Geometry: final body of the model. Coordinates: model frame, mm. A direction names the side the tool comes from. Give positions to 0.01 mm unless a question says otherwise; leave off trailing zeros. Write each loop counter-clockwise with the first axis right and the second up, starting at its lowest first coordinate (ties: lowest second). Pieces come first, ordered by that corner, then holes. Notation, with made-up numbers: M -7.75,71 L 42.25,71 A9 ccw 42.25,88 Z; hole C -18.5,5 d10. An arc over 180 degrees is marked long. Use a Markdown table: item, result. Add a question column.
(1) Draft query along X for faces 1 (the flat face through (24, 0, -25)), 2 (the flat face through (24, 14, -58)), 3 (the flat face through (-10, 13, -26)). Return one class per face: released by +X, released by -X, zero draft, split by the parting line, or undercut.
(2) Cut plane A-A (y = 24). Output: boundary loops of the cut face in (x, z), plus the area to 3 significant figures.
(3) Reachability of faces 4 (the flat face through (24, 13, -59)), 5 (the flat face through (23, 14, 7)) from +Z, -Z, +X, -X, +Y, -Y: full face, straight path, thin tool, end or side. Return the list, or none.
(4) Material intervals for L1, parallel to X at y = 4.5, z = -4.5; L2, parallel to Z at x = 45, y = 18; L3, parallel to Y at x = 19.5, z = -28, sorted ascending.
(5) Cut plane B-B (x = 29.5). Output: boundary loops of the cut face in (y, z), plus the area to 3 significant figures.
(6) Cut plane D-D (z = -8). Output: boundary loops of the cut face in (x, y), plus the area to 3 significant figures.
(7) Cut plane C-C (x = -3). Output: boundary loops of the cut face in (y, z), plus the area to 3 significant figures.
Autodesk Inventor part; units mm, degrees
ref_plane "YZ Plane" through (0, 0, 0) normal (1, 0, 0) x (0, 1, 0)
ref_plane "XZ Plane" through (0, 0, 0) normal (0, 1, 0) x (-1, 0, 0)
ref_plane "XY Plane" through (0, 0, 0) normal (0, 0, 1) x (1, 0, 0)
sketch "Boceto1" plane through (0, 0, 0) normal (0, 1, 0) x (-1, 0, 0)
  line L0 (9, 7) -> (-56, 7)
  line L1 (-56, 7) -> (-56, -58)
  line L2 (-56, -58) -> (9, -58)
  line L3 (9, -58) -> (9, 7)
  point P0 (0, 0)
  dimension "d0" = 65
  dimension "d1" = 65
extrude "Extrusión1" add sketch "Boceto1" along normal blind 3
sketch "Boceto2" plane through (0, 3, 0) normal (0, 1, 0) x (1, 0, 0)
  line L0 (-9, -7) -> (56, -7)
  line L1 (56, -7) -> (56, 58)
  line L2 (56, 58) -> (-9, 58)
  line L3 (-9, 58) -> (-9, -7)
  line L4 (-10, -8) -> (57, -8)
  line L5 (57, -8) -> (57, 59)
  line L6 (57, 59) -> (-10, 59)
  line L7 (-10, 59) -> (-10, -8)
  line L8 (-10, -8) -> (57, 59) construction
  line L9 (57, -8) -> (-10, 59) construction
  point P0 (0, 0)
  point P1 (23.5, 25.5)
  dimension "d4" = 67
  dimension "d5" = 67
extrude "Extrusión2" add sketch "Boceto2" against normal blind 3
sketch "Boceto3" plane through (0, 3, 0) normal (0, 1, 0) x (1, 0, 0)
  line L0 (-10, -8) -> (57, -8)
  line L1 (57, -8) -> (57, 59)
  line L2 (57, 59) -> (-10, 59)
  line L3 (-10, 59) -> (-10, -8)
  line L4 (-9, -7) -> (56, -7)
  line L5 (56, -7) -> (56, 58)
  line L6 (56, 58) -> (-9, 58)
  line L7 (-9, 58) -> (-9, -7)
  line L8 (-9, -7) -> (56, 58) construction
  line L9 (56, -7) -> (-9, 58) construction
  point P0 (0, 0)
  point P1 (23.5, 25.5)
  dimension "d8" = 65
  dimension "d9" = 65
extrude "Extrusión3" add sketch "Boceto3" along normal blind 23
sketch "Boceto4" plane through (-10, 0, 8) normal (0, 0, 1) x (1, 0, 0)
  line L0 (0, 26) -> (0, 0)
  line L1 (67, 0) -> (0, 0)
  line L2 (67, 0) -> (67, 26)
  line L3 (0, 26) -> (67, 26)
  line L4 (41, 9) -> (26, 9)
  line L5 (26, 9) -> (26, 5)
  line L6 (26, 5) -> (41, 5)
  line L7 (41, 5) -> (41, 9)
  line L8 (41, 9) -> (26, 5) construction
  line L9 (26, 9) -> (41, 5) construction
  point P0 (10, 0)
  point P1 (33.5, 7)
extrude "Extrusión4" cut sketch "Boceto4" against normal blind 50 contours L7 L6 L5 L4
sketch "Boceto6" plane through (0, 26, 0) normal (0, 1, 0) x (1, 0, 0)
  line L0 (57, 59) -> (-10, 59)
  line L1 (57, -8) -> (57, 59)
  line L2 (-10, -8) -> (57, -8)
  line L3 (-10, 59) -> (-10, -8)
  line L4 (-12.5, 61.5) -> (59.5, 61.5)
  line L5 (59.5, 61.5) -> (59.5, -10.5)
  line L6 (59.5, -10.5) -> (-12.5, -10.5)
  line L7 (-12.5, -10.5) -> (-12.5, 61.5)
  line L8 (-12.5, 61.5) -> (59.5, -10.5) construction
  line L9 (59.5, 61.5) -> (-12.5, -10.5) construction
  point P0 (0, 0)
  point P1 (23.5, 25.5)
  dimension "d14" = 72
  dimension "d15" = 72
properties part number "Cajapotenciometro_v1"
Answer list:
| question | item | result |
|---|---|---|
| 1 | face 1 | zero draft |
| 1 | face 2 | undercut |
| 1 | face 3 | released by -X |
| 2 | outline | M -10,-59 L 57,-59 L 57,8 L -10,8 Z; hole M -9,-58 L 56,-58 L 56,7 L -9,7 Z |
| 2 | area | 264 mm² |
| 3 | face 4 | -Z, +X, -X, +Y, -Y |
| 3 | face 5 | +Y |
| 4 | L1 | -10 to -9, 56 to 57 |
| 4 | L2 | -59 to -58, 7 to 8 |
| 4 | L3 | 0 to 3 |
| 5 | outline | M 0,-59 L 26,-59 L 26,-58 L 3,-58 L 3,7 L 5,7 L 5,8 L 0,8 Z; M 9,7 L 26,7 L 26,8 L 9,8 Z |
| 5 | area | 243 mm² |
| 6 | outline | M -10,0 L 57,0 L 57,26 L 56,26 L 56,3 L -9,3 L -9,26 L -10,26 Z |
| 6 | area | 247 mm² |
| 7 | outline | M 0,-59 L 26,-59 L 26,-58 L 3,-58 L 3,7 L 26,7 L 26,8 L 0,8 Z |
| 7 | area | 247 mm² |
